Check sheet for the modelled part. Datum: model origin and axes. Units: mm. A direction names the side the tool comes from. Round coordinates to 2 decimals unless told otherwise and drop trailing zeros. Order: outer loops, then holes, each group sorted by start corner. A loop starts at its lowest first (then second) coordinate and runs counter-clockwise, first axis right, second up.
(1) Sectioned sample at D-D, the plane z = 76. Enter the section's corners in (x, y), and give its area (3 significant figures).
(2) Sectioned sample at B-B, the plane x = 103. Enter the section's corners in (y, z), and give its area (3 significant figures).
(3) Mould release check, pull along X, two halves, no side actions. Record for faces 1 (the flat face through (197.2, -44.02, 274.65)), 2 (the flat face through (370, 335, -187)), 3 (the flat face through (400, 114, 7)): released by +X, released by -X, zero draft, split by the parting line, or undercut.
(4) Depth check by flat-ended pin: pin 1 (1 mm diameter, centred on x = 201, z = 385.5, fed in from +Y); pin 2 (5 mm diameter, centred on x = 81, y = 235, fed in from +Z); pin 3 (4 mm diameter, centred on x = 120, z = 220.5, fed in from -Y). Enter the tip coordinate at first touch or a pass-through.
(5) Thickness scan on probe 1 along X at (y, z) = (14.5, -116.5); probe 2 along Z at (x, y) = (250, 310); probe 3 along Y at (x, z) = (181, 279). Record the ranges inside material, lowest first.
(6) Sectioned sample at A-A, the plane z = -131.5. Enter the section's corners in (x, y).
(7) Sectioned sample at C-C, the plane y = 44. Enter the section's corners in (x, z).
(8) Tool access check on faces 4 (the flat face through (15, 320, -187)), 5 (the flat face through (169, 0, 3)), 6 (the flat face through (370, 15, -187)). Record the directions out of +Z, -Z, +X, -X, +Y, -Y that give a thin tool (end or side, any length) a straight path to the whole face; none if there is none.
```python
from build123d import *

# Parameters (mm, degrees)
F0_W     = 400
F0_H     = 350
F1_DEPTH = 25
F2_W     = 30
F2_H     = 30
F3_DEPTH = 380
F5_DEPTH = 400


with BuildPart() as f1:
    # F0 (on Top) → F1 (new body)
    with BuildSketch(Plane.XY):
        with Locations((200, 175)):
            Rectangle(F0_W, F0_H)
    extrude(amount=F1_DEPTH)

    # F2 (on face) → F3 (join)
    with BuildSketch(Plane(origin=(0, 0, 0), x_dir=(1, 0, 0), z_dir=(0, 0, -1))):
        with Locations((15, -15)):
            Rectangle(F2_W, F2_H)
        with Locations((385, -15)):
            Rectangle(F2_W, F2_H)
        with Locations((15, -335)):
            Rectangle(F2_W, F2_H)
        with Locations((385, -335)):
            Rectangle(F2_W, F2_H)
    extrude(amount=F3_DEPTH)

    # F4 (on Right) → F5 (join, through all)
    with BuildSketch(Plane.YZ):
        Polygon((-86.824089, 517.403877), (0, 25), (30.462798, 25), (-57.279856, 522.613322), align=None)
    extrude(amount=F5_DEPTH)


solid = f1.part
```
Derived:
1. outline: (0, -8.99) - (400, -8.99) - (400, 21.47) - (0, 21.47) - close
1. area: 12,200 mm2
2. outline: (-86.82, 517.4) - (0, 25) - (0, 0) - (350, 0) - (350, 25) - (30.46, 25) - (-57.28, 522.61) - close
2. area: 23,800 mm2
3. face 1: zero draft
3. face 2: undercut
3. face 3: released by +X
4. pin 1: stops at y = -33.01
4. pin 2: stops at z = 25
4. pin 3: stops at y = -34.82
5. probe 1: x = 0 to 30, 370 to 400
5. probe 2: z = 0 to 25
5. probe 3: y = -44.79 to -14.32
6. outline: (0, 0) - (30, 0) - (30, 30) - (0, 30) - close; (0, 320) - (30, 320) - (30, 350) - (0, 350) - close; (370, 0) - (400, 0) - (400, 30) - (370, 30) - close; (370, 320) - (400, 320) - (400, 350) - (370, 350) - close
7. outline: (0, 0) - (400, 0) - (400, 25) - (0, 25) - close
8. face 4: -Z, +X, -X
8. face 5: -Z, +X, -X, -Y
8. face 6: -Z, +Y, -Y
